Autodesk Inventor part; units mm, degrees
ref_plane "YZ Plane" through (0, 0, 0) normal (1, 0, 0) x (0, 1, 0)
ref_plane "XZ Plane" through (0, 0, 0) normal (0, 1, 0) x (-1, 0, 0)
ref_plane "XY Plane" through (0, 0, 0) normal (0, 0, 1) x (1, 0, 0)
sketch "Sketch1" plane through (0, 0, 0) normal (0, 1, 0) x (-1, 0, 0)
  line L0 (30, 45) -> (-30, 45)
  line L1 (-30, 45) -> (-30, -45)
  line L2 (-30, -45) -> (30, -45)
  line L3 (30, -45) -> (30, 45)
  line L4 (30, 45) -> (12.5, 45)
  line L5 (12.5, 45) -> (12.5, 85)
  line L6 (12.5, 85) -> (30, 85)
  line L7 (30, 85) -> (30, 45)
  line L8 (-30, 45) -> (-12.5, 45)
  line L9 (-12.5, 45) -> (-12.5, 85)
  line L10 (-12.5, 85) -> (-30, 85)
  line L11 (-30, 85) -> (-30, 45)
  line L12 (3.75, 45) -> (-3.75, 45)
  line L13 (-3.75, 45) -> (-3.75, 85)
  line L14 (-3.75, 85) -> (3.75, 85)
  line L15 (3.75, 85) -> (3.75, 45)
  point P0 (0, 0)
  point P1 (0, 45)
  dimension "d0" = 90
  dimension "d1" = 60
  dimension "d2" = 45
  dimension "d3" = 30
  dimension "d23" = 40
  dimension "d24" = 25
  dimension "d25" = 17.5
  dimension "d39" = 7.5
  dimension "d40" = 40
  dimension "d41" = 3.75
extrude "Extrusion1" add sketch "Sketch1" along normal blind 5
sketch "Sketch2" plane through (0, 5, 0) normal (0, 1, 0) x (1, 0, 0)
  line L0 (-24.5, -37.5) -> (24.5, -37.5)
  line L1 (24.5, -37.5) -> (24.5, 20.5)
  line L2 (24.5, 20.5) -> (-24.5, 20.5)
  line L3 (-24.5, 20.5) -> (-24.5, -37.5)
  line L4 (-12.5, -45) -> (12.5, -45)
  circle A0 centre (-24.5, -37.5) radius 1.35
  line L5 (-24.5, -8.5) -> (24.5, -8.5)
  line L6 (0, -37.5) -> (0, 20.5)
  circle A1 centre (24.5, -37.5) radius 1.35
  circle A2 centre (-24.5, 20.5) radius 1.35
  circle A3 centre (24.5, 20.5) radius 1.35
  point P0 (0, 0)
  point P1 (-30, -45)
  point P2 (30, -45)
  dimension "d6" = 49
  dimension "d7" = 58
  dimension "d8" = 24.5
  dimension "d9" = 7.5
  dimension "d10" = 2.7
  dimension "d13" = 49
  dimension "d16" = 58
extrude "Extrusion2" add sketch "Sketch2" along normal blind 5 contours L3 A0 L0 | L0 A0 L3 | A1 L1 L0 | L0 L1 A1 | A2 L2 L3 | L3 L2 A2 | A3 L2 L1 | L1 L2 A3
sketch "Sketch4" plane through (0, 0, 0) normal (1, 0, 0) x (0, 1, 0)
  line L0 (0, -45) -> (5, -45)
  line L1 (0, -45) -> (-16.853, -30.8587)
  line L2 (-16.853, -30.8587) -> (-15.246, -28.9436)
  line L3 (-15.246, -28.9436) -> (0, -41.7365)
  line L4 (0, -45) -> (0, 85)
  point P0 (0, 0)
  dimension "d28" = 130
  dimension "d29" = 2.5
  dimension "d30" = 22
extrude "Extrusion4" add sketch "Sketch4" along normal mid plane 25
sketch "Sketch6" plane through (12.5, 0, -45) normal (0, -0.6428, -0.766) x (-1, 0, 0)
  line L0 (-17.5, 0) -> (0, 0)
  line L1 (25, -22) -> (0, -22)
  line L2 (0, 0) -> (25, 0)
  line L3 (25, 0) -> (25, -22)
  line L4 (25, -22) -> (0, -22)
  line L5 (0, -22) -> (0, 0)
  line L6 (25, -2.0977) -> (0, -2.0977)
  circle A0 centre (2, -5.638) radius 1.1
  circle A1 centre (23, -5.638) radius 1.1
  circle A2 centre (2, -18.138) radius 1.1
  circle A3 centre (23, -18.138) radius 1.1
  line L7 (8.25, -13.788) -> (16.75, -13.788)
  line L8 (16.75, -13.788) -> (16.75, -22.288)
  line L9 (16.75, -22.288) -> (8.25, -22.288)
  line L10 (8.25, -22.288) -> (8.25, -13.788)
  line L11 (0, -22) -> (0, 0)
  line L12 (25, -22) -> (25, -2.0977)
  line L13 (0, -3.638) -> (25, -3.638)
  line L14 (25, -3.638) -> (25, -27.5)
  line L15 (25, -27.5) -> (0, -27.5)
  line L16 (0, -27.5) -> (0, -3.638)
  line L17 (12.5, -13.788) -> (12.5, -22.288)
  line L18 (8.25, -18.038) -> (16.75, -18.038)
  dimension "d42" = 2.2
  dimension "d43" = 2.2
  dimension "d44" = 2.2
  dimension "d45" = 2.2
  dimension "d47" = 2
  dimension "d48" = 0
  dimension "d50" = 0
  dimension "d52" = 0
  dimension "d53" = 2
  dimension "d56" = 0
  dimension "d59" = 12.5
  dimension "d60" = 8.5
  dimension "d61" = 8.5
  dimension "d63" = 23.862
  dimension "d65" = 2
  dimension "d66" = 12.5
  dimension "d69" = 9.462
  dimension "d70" = 5.5
extrude "Extrusion5" cut sketch "Sketch6" against normal blind 5 contours A0 | A1 | A2 | A3
sketch "Sketch9" plane through (12.5, 0, -45) normal (0, -0.6428, -0.766) x (-1, 0, 0)
  circle A0 centre (12.5, -18.038) radius 0.2236
  point P0 (12.5, -28.9254)
properties part number "Platform"
Input: part model. Units: mm. Frame: model coordinates. A direction names the side the tool comes from. Round coordinates to 2 decimals unless told otherwise and drop trailing zeros. Loops run counter-clockwise (first coordinate to the right, second up) from the corner with the lowest first, then second, coordinate; pieces in that order, holes last. Notation, with made-up numbers: M 50,55.5 L 75,55.5 A20 cw 75,74.5 Z; hole C 5,-4 d11. An arc over 180 degrees is marked long. Answer as CSV lines item,"result". Start each with the question number.
(1) Section B-B, the plane z = -20.5. Output: boundary loops of the cut face in (x, y), plus the area to 3 significant figures.
(2) Line query: line 1 (X direction, y = 1, z = 48.5); line 2 (Y direction, x = 18, z = 78.5); line 3 (X direction, y = -4.75, z = -38). Output: solid intervals per line, ascending. Write a range as [from, to].
(3) Reachability of faces 4 (the cylindrical face through (-11.516, -3.849, -40.161)), 5 (the flat face through (12.5, -8, -36)), 6 (the flat face through (12.5, 2, 65)), 7 (the flat face through (-25, 10, -21)), 8 (the cylindrical face through (25.747, 7.465, -21.017)) from +Z, -Z, +X, -X, +Y, -Y: full face, straight path, thin tool, end or side. Return the list, or none.
(4) Section D-D, the plane z = 6.5. Output: boundary loops of the cut face in (x, y).
(5) Section A-A, the plane x = 24.5. Output: boundary loops of the cut face in (y, z).
(6) Draft query along X for faces 1 (the flat face through (-12.5, -8, -36)), 2 (the flat face through (-12.5, 2, 65)), 3 (the flat face through (-0.175, -8.309, -38.028)). Return one class per face: released by +X, released by -X, zero draft, split by the parting line, or undercut.
(7) Section C-C, the plane x = 2. Output: boundary loops of the cut face in (y, z), plus the area to 3 significant figures.
(8) First-contact query: pin 1 (3 mm diameter, centred on y = -0.5, z = -16.5, fed in from -X); pin 2 (8 mm diameter, centred on y = -11.5, z = -35, fed in from -X); pin 3 (5 mm diameter, centred on x = 13, z = 57, fed in from -Y); pin 4 (4 mm diameter, centred on x = 9, y = 2.5, fed in from +Z). Flat tips, straight axial feed; report the tip coordinate or a pass-through.
Values found:
1,outline,"M -30,0 L 30,0 L 30,5 L 25.85,5 L 25.85,10 L 23.15,10 L 23.15,5 L -23.15,5 L -23.15,10 L -25.85,10 L -25.85,5 L -30,5 Z"
1,area,"327 mm²"
2,line 1,"x = [-30, -12.5], [-3.75, 3.75], [12.5, 30]"
2,line 2,"y = [0, 5]"
2,line 3,"x = [-12.5, 12.5]"
3,face 4,"none"
3,face 5,"+Z, -Z, +X, -Y"
3,face 6,"+Z, +Y, -Y"
3,face 7,"+Z, -Z, +X, -X, +Y"
3,face 8,"+Y"
4,outline,"M -30,0 L 30,0 L 30,5 L -30,5 Z"
5,outline,"M 0,-45 L 5,-45 L 5,-21.85 L 10,-21.85 L 10,-19.15 L 5,-19.15 L 5,36.15 L 10,36.15 L 10,38.85 L 5,38.85 L 5,85 L 0,85 Z"
6,face 1,"released by -X"
6,face 2,"undercut"
6,face 3,"zero draft"
7,outline,"M -16.85,-30.86 L 0,-45 L 5,-45 L 5,85 L 0,85 L 0,-41.74 L -15.25,-28.94 Z"
7,area,"702 mm²"
8,pin 1,"stops at x = -30"
8,pin 2,"stops at x = -12.5"
8,pin 3,"stops at y = 0"
8,pin 4,"stops at z = 45"
